from build123d import *
from OCP.BRepFilletAPI import BRepFilletAPI_MakeChamfer

# Parameters (mm, degrees)
SKETCH1_R               = 9.85
SKETCH1_R_2             = 0.675
BOSS_EXTRUDE1_DEPTH     = 14.5
BOSS_EXTRUDE2_DEPTH     = 16
BOSS_EXTRUDE3_START     = 14.5
SKETCH1_4_R             = 9.85
SKETCH1_4_R_2           = 0.675
BOSS_EXTRUDE3_DEPTH     = 4.9
BOSS_EXTRUDE4_START     = -17.65
SKETCH1_5_R             = 9.85
SKETCH1_5_R_2           = 0.675
BOSS_EXTRUDE4_DEPTH     = 3.15
BOSS_EXTRUDE5_START     = 1.05
BOSS_EXTRUDE5_DEPTH     = 1.05
SKETCH3_W               = 18.5
SKETCH3_H               = 13.5
BOSS_EXTRUDE6_DEPTH     = 1.85
CHAMFER1_SIZE           = 2.1
CHAMFER1_SIZE2          = 1.762109225
BOSS_EXTRUDE7_DEPTH     = 1.5
CUT_EXTRUDE1_START      = 16
SKETCH4_R               = 0.925
CUT_EXTRUDE1_DEPTH      = 5
CUT_EXTRUDE2_START      = -11
SKETCH4_3_R             = 0.925
CUT_EXTRUDE2_DEPTH      = 5
CHAMFER2_SIZE           = 2
CHAMFER2_SIZE2          = 1.678199262
CHAMFER3_SIZE           = 0.5
CHAMFER3_SIZE2          = 0.419549816
BOSS_EXTRUDE8_START     = 19.4
SKETCH5_R               = 3.875
BOSS_EXTRUDE8_DEPTH     = 0.5
BOSS_EXTRUDE9_START     = -18.2
SKETCH5_2_R             = 3.875
BOSS_EXTRUDE9_DEPTH     = 0.55
CUT_EXTRUDE3_DEPTH      = 43.196474971
CUT_EXTRUDE3_DEPTH_BACK = 43.196474971
SKETCH6_R               = 1.375


with BuildPart() as part:
    # Sketch1 → Boss-Extrude1 (new, symmetric)
    # profile 1 of 11: a face of its own
    with BuildSketch(Plane.XY):
        with BuildLine():
            Line((-12.35, 10.1), (-12.35, -5.794609564))
            Line((-12.35, -5.794609564), (-9.35, -5.794609564))
            ThreePointArc((-9.35, -5.794609564), (0, -11), (9.35, -5.794609564))
            Line((9.35, -5.794609564), (12.35, -5.794609564))
            Line((12.35, -5.794609564), (12.35, 10.1))
            Line((12.35, 10.1), (-12.35, 10.1))
        make_face()
        Circle(SKETCH1_R, mode=Mode.SUBTRACT)
    # profile 2 of 11: a face of its own
    with BuildSketch(Plane.XY):
        Circle(SKETCH1_R)
        with Locations((-4.949747468, 4.949747468)):
            Circle(SKETCH1_R_2, mode=Mode.SUBTRACT)
        with Locations((-7, 0)):
            Circle(SKETCH1_R_2, mode=Mode.SUBTRACT)
        with Locations((-4.949747468, -4.949747468)):
            Circle(SKETCH1_R_2, mode=Mode.SUBTRACT)
        with Locations((0, -7)):
            Circle(SKETCH1_R_2, mode=Mode.SUBTRACT)
        with Locations((4.949747468, -4.949747468)):
            Circle(SKETCH1_R_2, mode=Mode.SUBTRACT)
        with Locations((7, 0)):
            Circle(SKETCH1_R_2, mode=Mode.SUBTRACT)
        with Locations((4.949747468, 4.949747468)):
            Circle(SKETCH1_R_2, mode=Mode.SUBTRACT)
        with Locations((0, 7)):
            Circle(SKETCH1_R_2, mode=Mode.SUBTRACT)
    # profile 3 of 11: a face of its own
    with BuildSketch(Plane.XY):
        with Locations((-4.949747468, 4.949747468)):
            Circle(SKETCH1_R_2)
    # profile 4 of 11: a face of its own
    with BuildSketch(Plane.XY):
        with Locations((-7, 0)):
            Circle(SKETCH1_R_2)
    # profile 5 of 11: a face of its own
    with BuildSketch(Plane.XY):
        with Locations((-4.949747468, -4.949747468)):
            Circle(SKETCH1_R_2)
    # profile 6 of 11: a face of its own
    with BuildSketch(Plane.XY):
        with Locations((0, -7)):
            Circle(SKETCH1_R_2)
    # profile 7 of 11: a face of its own
    with BuildSketch(Plane.XY):
        with Locations((4.949747468, -4.949747468)):
            Circle(SKETCH1_R_2)
    # profile 8 of 11: a face of its own
    with BuildSketch(Plane.XY):
        with Locations((7, 0)):
            Circle(SKETCH1_R_2)
    # profile 9 of 11: a face of its own
    with BuildSketch(Plane.XY):
        with Locations((4.949747468, 4.949747468)):
            Circle(SKETCH1_R_2)
    # profile 10 of 11: a face of its own
    with BuildSketch(Plane.XY):
        with Locations((0, 7)):
            Circle(SKETCH1_R_2)
    # profile 11 of 11: a face of its own
    with BuildSketch(Plane.XY):
        with BuildLine():
            Line((-9.35, -5.794609564), (-12.35, -5.794609564))
            Line((-12.35, -5.794609564), (-12.35, -35.1))
            Line((-12.35, -35.1), (12.35, -35.1))
            Line((12.35, -35.1), (12.35, -5.794609564))
            Line((12.35, -5.794609564), (9.35, -5.794609564))
            ThreePointArc((9.35, -5.794609564), (0, -11), (-9.35, -5.794609564))
        make_face()
    extrude(amount=BOSS_EXTRUDE1_DEPTH, both=True)

    # Sketch1<3> → Boss-Extrude2 (add, symmetric)
    with BuildSketch(Plane.XY):
        with BuildLine():
            Line((-9.35, -5.794609564), (-12.35, -5.794609564))
            Line((-12.35, -5.794609564), (-12.35, -35.1))
            Line((-12.35, -35.1), (12.35, -35.1))
            Line((12.35, -35.1), (12.35, -5.794609564))
            Line((12.35, -5.794609564), (9.35, -5.794609564))
            ThreePointArc((9.35, -5.794609564), (0, -11), (-9.35, -5.794609564))
        make_face()
    extrude(amount=BOSS_EXTRUDE2_DEPTH, both=True)

    # Sketch1<4> → Boss-Extrude3 (add)
    with BuildSketch(Plane.XY.offset(BOSS_EXTRUDE3_START)):
        Circle(SKETCH1_4_R)
        with Locations((0, 7)):
            Circle(SKETCH1_4_R_2, mode=Mode.SUBTRACT)
        with Locations((4.949747468, 4.949747468)):
            Circle(SKETCH1_4_R_2, mode=Mode.SUBTRACT)
        with Locations((7, 0)):
            Circle(SKETCH1_4_R_2, mode=Mode.SUBTRACT)
        with Locations((4.949747468, -4.949747468)):
            Circle(SKETCH1_4_R_2, mode=Mode.SUBTRACT)
        with Locations((0, -7)):
            Circle(SKETCH1_4_R_2, mode=Mode.SUBTRACT)
        with Locations((-4.949747468, -4.949747468)):
            Circle(SKETCH1_4_R_2, mode=Mode.SUBTRACT)
        with Locations((-7, 0)):
            Circle(SKETCH1_4_R_2, mode=Mode.SUBTRACT)
        with Locations((-4.949747468, 4.949747468)):
            Circle(SKETCH1_4_R_2, mode=Mode.SUBTRACT)
    extrude(amount=BOSS_EXTRUDE3_DEPTH)

    # Sketch1<5> → Boss-Extrude4 (add)
    with BuildSketch(Plane.XY.offset(BOSS_EXTRUDE4_START)):
        Circle(SKETCH1_5_R)
        with Locations((0, 7)):
            Circle(SKETCH1_5_R_2, mode=Mode.SUBTRACT)
        with Locations((4.949747468, 4.949747468)):
            Circle(SKETCH1_5_R_2, mode=Mode.SUBTRACT)
        with Locations((7, 0)):
            Circle(SKETCH1_5_R_2, mode=Mode.SUBTRACT)
        with Locations((4.949747468, -4.949747468)):
            Circle(SKETCH1_5_R_2, mode=Mode.SUBTRACT)
        with Locations((0, -7)):
            Circle(SKETCH1_5_R_2, mode=Mode.SUBTRACT)
        with Locations((-4.949747468, -4.949747468)):
            Circle(SKETCH1_5_R_2, mode=Mode.SUBTRACT)
        with Locations((-7, 0)):
            Circle(SKETCH1_5_R_2, mode=Mode.SUBTRACT)
        with Locations((-4.949747468, 4.949747468)):
            Circle(SKETCH1_5_R_2, mode=Mode.SUBTRACT)
    extrude(amount=BOSS_EXTRUDE4_DEPTH)

    # Sketch2 → Boss-Extrude5 (add)
    with BuildSketch(Plane.XY.offset(16).offset(BOSS_EXTRUDE5_START)):
        with BuildLine():
            Line((-7, -8.485281374), (-7, -35.1))
            Line((-7, -35.1), (7, -35.1))
            Line((7, -35.1), (7, -8.485281374))
            ThreePointArc((7, -8.485281374), (0, -11), (-7, -8.485281374))
        make_face()
    extrude(amount=-BOSS_EXTRUDE5_DEPTH)

    # Sketch3 → Boss-Extrude6 (add)
    with BuildSketch(Plane(origin=(0, 0, -16), x_dir=(-1, 0, 0), z_dir=(0, 0, -1))):
        with Locations((0, -23.75)):
            Rectangle(SKETCH3_W, SKETCH3_H)
    extrude(amount=BOSS_EXTRUDE6_DEPTH)

    # Chamfer1
    chamfer1_edges = [part.edges().sort_by_distance(p)[0] for p in [
        (0, -17, -17.85),
    ]]
    chamfer1_side = [part.faces().sort_by_distance(p)[0] for p in [
        (0, -23.75, -17.85),
    ]]
    chamfer(chamfer1_edges, length=CHAMFER1_SIZE, length2=CHAMFER1_SIZE2, reference=chamfer1_side[0])

    # Sketch3<3> → Boss-Extrude7 (add)
    with BuildSketch(Plane(origin=(0, 0, -16), x_dir=(-1, 0, 0), z_dir=(0, 0, -1))):
        Polygon((-10, -17), (-9.25, -17), (9.25, -17), (10, -17), (10, -12), (-10, -12), align=None)
    extrude(amount=BOSS_EXTRUDE7_DEPTH)

    # Sketch4 → Cut-Extrude1 (cut)
    with BuildSketch(Plane.XY.offset(CUT_EXTRUDE1_START)):
        with Locations((-10.5, -8.5)):
            Circle(SKETCH4_R)
        with Locations((10.5, -8.5)):
            Circle(SKETCH4_R)
        with Locations((-10.5, -29.5)):
            Circle(SKETCH4_R)
        with Locations((10.5, -29.5)):
            Circle(SKETCH4_R)
    extrude(amount=-CUT_EXTRUDE1_DEPTH, mode=Mode.SUBTRACT)

    # Sketch4<3> → Cut-Extrude2 (cut)
    with BuildSketch(Plane.XY.offset(CUT_EXTRUDE2_START)):
        with Locations((10.5, -8.5)):
            Circle(SKETCH4_3_R)
        with Locations((-10.5, -8.5)):
            Circle(SKETCH4_3_R)
        with Locations((-10.5, -33)):
            Circle(SKETCH4_3_R)
        with Locations((10.5, -33)):
            Circle(SKETCH4_3_R)
    extrude(amount=-CUT_EXTRUDE2_DEPTH, mode=Mode.SUBTRACT)

    # Chamfer2: one chamfer whose edges measure the first distance from different faces: ONE call of the kernel's chamfer builder (chamfer() names one face for all edges)
    chamfer2_edges_1 = [part.edges().sort_by_distance(p)[0] for p in [
        (-12.35, 10.1, 0),
    ]]
    chamfer2_side_1 = [part.faces().sort_by_distance(p)[0] for p in [
        (0, 10.1, 0),
    ]]
    chamfer2_edges_2 = [part.edges().sort_by_distance(p)[0] for p in [
        (12.35, 10.1, 0),
    ]]
    chamfer2_side_2 = [part.faces().sort_by_distance(p)[0] for p in [
        (12.35, -12.999527083, 0),
    ]]
    chamfer2 = BRepFilletAPI_MakeChamfer(part.part.solid().wrapped)
    for e in chamfer2_edges_1:
        chamfer2.Add(CHAMFER2_SIZE, CHAMFER2_SIZE2, e.wrapped, chamfer2_side_1[0].wrapped)  # the first distance lies on this face
    for e in chamfer2_edges_2:
        chamfer2.Add(CHAMFER2_SIZE, CHAMFER2_SIZE2, e.wrapped, chamfer2_side_2[0].wrapped)  # the first distance lies on this face
    add(Compound.cast(chamfer2.Shape()), mode=Mode.REPLACE)

    # Chamfer3: one chamfer whose edges measure the first distance from different faces: ONE call of the kernel's chamfer builder (chamfer() names one face for all edges)
    chamfer3_edges_1 = [part.edges().sort_by_distance(p)[0] for p in [
        (12.35, -20.447304782, -16),
    ]]
    chamfer3_side_1 = [part.faces().sort_by_distance(p)[0] for p in [
        (10.85, -6.177871343, -16),
    ]]
    chamfer3_edges_2 = [part.edges().sort_by_distance(p)[0] for p in [
        (-12.35, -20.447304782, 16),
    ]]
    chamfer3_side_2 = [part.faces().sort_by_distance(p)[0] for p in [
        (-9.6888762, -20.825200729, 16),
    ]]
    chamfer3_edges_3 = [part.edges().sort_by_distance(p)[0] for p in [
        (12.35, -20.447304782, 16),
    ]]
    chamfer3_side_3 = [part.faces().sort_by_distance(p)[0] for p in [
        (12.35, -13.955562818, 0),
    ]]
    chamfer3_edges_4 = [part.edges().sort_by_distance(p)[0] for p in [
        (-12.35, -20.447304782, -16),
    ]]
    chamfer3_side_4 = [part.faces().sort_by_distance(p)[0] for p in [
        (-12.35, -13.801991321, 0),
    ]]
    chamfer3 = BRepFilletAPI_MakeChamfer(part.part.solid().wrapped)
    for e in chamfer3_edges_1:
        chamfer3.Add(CHAMFER3_SIZE, CHAMFER3_SIZE2, e.wrapped, chamfer3_side_1[0].wrapped)  # the first distance lies on this face
    for e in chamfer3_edges_2:
        chamfer3.Add(CHAMFER3_SIZE, CHAMFER3_SIZE2, e.wrapped, chamfer3_side_2[0].wrapped)  # the first distance lies on this face
    for e in chamfer3_edges_3:
        chamfer3.Add(CHAMFER3_SIZE, CHAMFER3_SIZE2, e.wrapped, chamfer3_side_3[0].wrapped)  # the first distance lies on this face
    for e in chamfer3_edges_4:
        chamfer3.Add(CHAMFER3_SIZE, CHAMFER3_SIZE2, e.wrapped, chamfer3_side_4[0].wrapped)  # the first distance lies on this face
    add(Compound.cast(chamfer3.Shape()), mode=Mode.REPLACE)

    # Sketch5 → Boss-Extrude8 (add)
    with BuildSketch(Plane.XY.offset(BOSS_EXTRUDE8_START)):
        Circle(SKETCH5_R)
    extrude(amount=BOSS_EXTRUDE8_DEPTH)

    # Sketch5<2> → Boss-Extrude9 (add)
    with BuildSketch(Plane.XY.offset(BOSS_EXTRUDE9_START)):
        Circle(SKETCH5_2_R)
    extrude(amount=BOSS_EXTRUDE9_DEPTH)

    # Sketch6 → Cut-Extrude3 (cut, two sides: drawn at the far end of the back side and taken through both)
    with BuildSketch(Plane.XY.offset(-CUT_EXTRUDE3_DEPTH_BACK)):
        Circle(SKETCH6_R)
    extrude(amount=CUT_EXTRUDE3_DEPTH + CUT_EXTRUDE3_DEPTH_BACK, mode=Mode.SUBTRACT)


solid = part.part
The model under review builds one solid part; all positions refer to its coordinate system, in mm. A direction names the side the tool comes from. Round coordinates to 2 decimals unless told otherwise and drop trailing zeros. Loops run counter-clockwise (first coordinate to the right, second up) from the corner with the lowest first, then second, coordinate; pieces in that order, holes last. Notation, with made-up numbers: M 74,6.5 L 127,6.5 A26 ccw 127,38.5 Z; hole C 35.5,42 d9. An arc over 180 degrees is marked long. Answer as CSV lines item,"result".
1. Insertion check: pin 1 Ø2 at (x, y) = (-4.95, -4.95) entering from -Z; pin 2 Ø2 at (x, y) = (-3, -11) entering from +Z; pin 3 Ø1.5 at (x, y) = (-0.5, -14.5) entering from -Z. Each pin has a flat end and moves straight along its axis. Give the tip position at first contact, or say it passes through.
Outcome:
pin 1,"stops at z = -17.65"
pin 2,"stops at z = 17.05"
pin 3,"stops at z = -17.5"
2. Draft analysis for pull direction Y (two halves, no side actions). For faces 1 (the face through (0, 10.1, 0)), 2 (the face through (-5, 5, -14.5)), 3 (the face through (-7, -21.6, 16.5)), 4 (the face through (-5, -5, -14.5)), state which applies: pulls with the +Y half, pulls with the -Y half, needs draft (parallel to the pull), parting line crosses it, or undercut.
Outcome:
face 1,"pulls with the +Y half"
face 2,"undercut"
face 3,"needs draft"
face 4,"undercut"
3. We need section A-A (y = -33). Give the boundary of the cut face in (x, z) (3 decimals).
Outcome:
outline,"M -12.35,-15.5 L -11.93,-16 L -11.425,-16 L -11.425,-11 L -9.575,-11 L -9.575,-16 L 9.575,-16 L 9.575,-11 L 11.425,-11 L 11.425,-16 L 11.85,-16 L 12.35,-15.58 L 12.35,15.5 L 11.93,16 L 7,16 L 7,17.05 L -7,17.05 L -7,16 L -11.85,16 L -12.35,15.58 Z"
4. We need section C-C (y = -13). Give the boundary of the cut face in (x, z), plus the area to 3 significant figures.
Outcome:
outline,"M -12.35,-15.5 L -11.93,-16 L -10,-16 L -10,-17.5 L 10,-17.5 L 10,-16 L 11.85,-16 L 12.35,-15.58 L 12.35,15.5 L 11.93,16 L 7,16 L 7,17.05 L -7,17.05 L -7,16 L -11.85,16 L -12.35,15.58 Z"
area,"835 mm2"
5. To check wall thickness, follow L1, parallel to X at y = -33, z = -13 (3 decimals); L2, parallel to Z at x = 7.5, y = -9.5; L3, parallel to Z at x = 3, y = -22.5. State the ranges of each line that lie inside material, in increasing order. Write a range as [from, to].
Outcome:
L1,"x = [-12.35, -11.425], [-9.575, 9.575], [11.425, 12.35]"
L2,"z = [-16, 16]"
L3,"z = [-17.85, 17.05]"
6. For faces 5 (the face through (-7.674, 0.03, 16.916)), 6 (the face through (-0.3, -1.34, 0.58)), 7 (the face through (-0.09, 7.67, -16.1)), 8 (the face through (0, -2, -18.2)), 9 (the face through (-11, -5.795, 15)), list the 3-axis set-ups (+Z, -Z, +X, -X, +Y, -Y) from which the entire face can be reached by the end or side of a thin tool; tool diameter is ignored.
Outcome:
face 5,"+Z"
face 6,"+Z, -Z"
face 7,"-Z"
face 8,"-Z, +X, -X, +Y, -Y"
face 9,"+Z, -X"
7. We need section D-D (y = -25.5). Give the boundary of the cut face in (x, z).
Outcome:
outline,"M -12.35,-15.5 L -11.93,-16 L -9.25,-16 L -9.25,-17.85 L 9.25,-17.85 L 9.25,-16 L 11.85,-16 L 12.35,-15.58 L 12.35,15.5 L 11.93,16 L 7,16 L 7,17.05 L -7,17.05 L -7,16 L -11.85,16 L -12.35,15.58 Z"
8. We need section B-B (x = -8.5). Give the boundary of the cut face in (y, z), plus the area to 3 significant figures.
Outcome:
outline,"M -35.1,-16 L -30.5,-16 L -30.5,-17.85 L -19.1,-17.85 L -17,-16.09 L -17,-17.5 L -12,-17.5 L -12,-16 L -6.98,-16 L -6.98,-14.5 L -4.98,-14.5 L -4.98,-17.65 L 4.98,-17.65 L 4.98,-14.5 L 10.1,-14.5 L 10.1,14.5 L 4.98,14.5 L 4.98,19.4 L -4.98,19.4 L -4.98,14.5 L -6.98,14.5 L -6.98,16 L -35.1,16 Z"
area,"1,510 mm2"
